Could you check a few things on this model? Use its own coordinates, in mm. Round coordinates to 2 decimals unless told otherwise and drop trailing zeros. Loops run counter-clockwise (first coordinate to the right, second up) from the corner with the lowest first, then second, coordinate; pieces in that order, holes last.
Autodesk Inventor part; units mm, degrees
ref_plane "YZ Plane" through (0, 0, 0) normal (1, 0, 0) x (0, 1, 0)
ref_plane "XZ Plane" through (0, 0, 0) normal (0, 1, 0) x (-1, 0, 0)
ref_plane "XY Plane" through (0, 0, 0) normal (0, 0, 1) x (1, 0, 0)
sketch "スケッチ3" plane through (0, 0, 0) normal (0, 0, 1) x (1, 0, 0)
  line L0 (60, -99.3436) -> (-60, -99.3436)
  line L1 (-60, -99.3436) -> (-60, 99.3436)
  line L2 (-60, 99.3436) -> (60, 99.3436)
  line L3 (60, 99.3436) -> (60, -99.3436)
  line L4 (60, -99.3436) -> (-60, 99.3436) construction
  line L5 (-60, -99.3436) -> (60, 99.3436) construction
  point P0 (0, 0)
  dimension "d25" = 120
extrude "押し出し1" add sketch "スケッチ3" against normal blind 3
sketch "スケッチ4" plane through (0, 0, 0) normal (0, 0, 1) x (1, 0, 0)
  line L0 (0, 45.0711) -> (68.3595, 45.0711)
  line L1 (68.3595, 45.0711) -> (-74.3824, 45.0711)
  line L2 (-74.3824, 45.0711) -> (108.1656, 45.0711)
  line L3 (108.1656, 45.0711) -> (108.1656, 129.4154)
  line L4 (108.1656, 129.4154) -> (-74.3824, 129.4154)
  line L5 (-74.3824, 129.4154) -> (-74.3824, 45.0711)
  point P0 (0, 0)
extrude "押し出し4" cut sketch "スケッチ4" against normal blind 10
sketch "スケッチ12" plane through (0, 0, 0) normal (0, 0, 1) x (1, 0, 0)
  circle A0 centre (0, 0) radius 7.5
  circle A1 centre (0, 0) radius 22.5
  dimension "d85" = 15
  dimension "d93" = 45
sketch "スケッチ13" plane through (0, 0, 0) normal (0, 0, 1) x (1, 0, 0)
  circle A0 centre (0, 0) radius 7.5
  circle A1 centre (0, 0) radius 32.5
  circle A2 centre (31.7707, 6.8465) radius 25
  circle A3 centre (31.7707, 6.8465) radius 7.5
  circle A4 centre (31.7707, 6.8465) radius 32.5
  circle A5 centre (28.5436, -25.4929) radius 25
  circle A6 centre (28.5436, -25.4929) radius 20
  circle A7 centre (28.5436, -25.4929) radius 60
  circle A8 centre (0, -78.2685) radius 40
  circle A9 centre (0, -78.2685) radius 50
  circle A10 centre (31.7707, 6.8465) radius 5
  circle A11 centre (28.5436, -25.4929) radius 9.5
  circle A12 centre (0, -78.2685) radius 9.5
  dimension "d87" = 65
  dimension "d89" = 65
  dimension "d91" = 120
  dimension "d86" = 15
  dimension "d88" = 15
  dimension "d90" = 40
  dimension "d92" = 100
  dimension "d96" = 10
  dimension "d97" = 19
  dimension "d98" = 19
extrude "押し出し15" cut sketch "スケッチ12" against normal blind 10 contours A0
extrude "押し出し16" cut sketch "スケッチ13" against normal blind 10 contours A10 A1 | A1 A10 | A11 A1 A2 | A2 A1 A4 A11 | A4 A1 A11 | A2 A11 A4 A1 | A1 A11 A2 | A4 A11 A1 | A12 A7 | A7 A12
sketch "スケッチ14" plane through (0, 0, 0) normal (0, 0, 1) x (1, 0, 0)
  line L0 (-60, -99.3436) -> (-60, 45.0711)
  line L1 (60, 45.0711) -> (60, -99.3436)
  line L2 (-60, 45.0711) -> (60, 45.0711)
  line L3 (60, 45.0711) -> (60, -92.9289)
  line L4 (60, -92.9289) -> (-60, -92.9289)
  line L5 (-60, -92.9289) -> (-60, 45.0711)
  point P0 (0, 0)
  dimension "d101" = 138
extrude "押し出し17" cut sketch "スケッチ14" against normal blind 10 keep common part
sketch "スケッチ15" plane through (-60, 45.0711, 0) normal (0, 1, 0) x (1, 0, 0)
  line L0 (-15.5399, 21.7204) -> (138.9638, 21.7204)
  line L1 (138.9638, 21.7204) -> (138.9638, -41.1938)
  line L2 (138.9638, -41.1938) -> (-15.5399, -41.1938)
  line L3 (-15.5399, -41.1938) -> (-15.5399, 21.7204)
  point P0 (60, 0)
extrude "押し出し18" cut sketch "スケッチ15" against normal blind 10
sketch "スケッチ16" plane through (0, 0, 0) normal (0, 0, 1) x (1, 0, 0)
  circle A0 centre (31.7707, 6.8465) radius 5
  circle A1 centre (31.7707, 6.8465) radius 25
  circle A2 centre (28.5436, -25.4929) radius 9.5
  circle A3 centre (28.5436, -25.4929) radius 25
  circle A4 centre (55, -13) radius 2
  circle A5 centre (-55, -13) radius 2
  circle A6 centre (0, 29) radius 2
  point P0 (0, 0)
  dimension "d109" = 50
  dimension "d110" = 50
  dimension "d111" = 4
  dimension "d112" = 4
  dimension "d113" = 4
extrude "押し出し19" cut sketch "スケッチ16" against normal blind 10 contours A4 | A5 | A6
sketch "スケッチ17" plane through (0, 0, 0) normal (0, 0, 1) x (1, 0, 0)
  line L0 (0, 0) -> (0, 14.5)
  line L1 (0, 14.5) -> (0, -14.5)
  circle A0 centre (0, 14.5) radius 2.15
  circle A1 centre (0, -14.5) radius 2.15
  dimension "d116" = 14.5
  dimension "d117" = 29
  dimension "d118" = 4.3
  dimension "d119" = 4.3
extrude "押し出し20" cut sketch "スケッチ17" against normal blind 10
properties part number "板2" material "アルミニウム 6061"
Item 1: If we section it at C-C, the plane x = 0: Please give me the cut outline in (y, z).
Results list:
outline: (-92.93, -3) - (-87.77, -3) - (-87.77, 0) - (-92.93, 0) - close; (-68.77, -3) - (-16.65, -3) - (-16.65, 0) - (-68.77, 0) - close; (-12.35, -3) - (-7.5, -3) - (-7.5, 0) - (-12.35, 0) - close; (7.5, -3) - (12.35, -3) - (12.35, 0) - (7.5, 0) - close; (16.65, -3) - (27, -3) - (27, 0) - (16.65, 0) - close; (31, -3) - (35.07, -3) - (35.07, 0) - (31, 0) - close
Item 2: We'd pull the mould along Y, two halves only. Please class faces 1 (the cylindrical face through (0, 27, -1)), 2 (the flat face through (60, -28, -1)), 3 (the flat face through (1, -92.929, -1)): released by +Y, released by -Y, zero draft, split by the parting line, or undercut.
Results list:
face 1: undercut
face 2: zero draft
face 3: released by -Y
Item 3: If we section it at D-D, the plane x = 29.5: Please give me the cut outline in (y, z), then the cut area to 3 significant figures.
Results list:
outline: (-92.93, -3) - (-34.94, -3) - (-34.94, 0) - (-92.93, 0) - close; (-16.04, -3) - (2.39, -3) - (2.39, 0) - (-16.04, 0) - close; (11.3, -3) - (35.07, -3) - (35.07, 0) - (11.3, 0) - close
area: 301 mm2
Item 4: If we section it at A-A, the plane y = 0: Please give me the cut outline in (x, z), then the cut area to 3 significant figures.
Results list:
outline: (-60, -3) - (-7.5, -3) - (-7.5, 0) - (-60, 0) - close; (7.5, -3) - (60, -3) - (60, 0) - (7.5, 0) - close
area: 315 mm2
Item 5: If we section it at B-B, the plane x = 55: Please give me the cut outline in (y, z), then the cut area to 3 significant figures.
Results list:
outline: (-92.93, -3) - (-15, -3) - (-15, 0) - (-92.93, 0) - close; (-11, -3) - (35.07, -3) - (35.07, 0) - (-11, 0) - close
area: 372 mm2
Item 6: If I drill on line 1 along Y through (x, z) = (0, -1.6); line 2 along Y through (x, z) = (-55, -2.25); line 3 along X through (y, z) = (-14.5, -1.6), over which ranges is the centre line in solid material (lowest first)?
Results list:
line 1: y = -92.93 to -87.77, -68.77 to -16.65, -12.35 to -7.5, 7.5 to 12.35, 16.65 to 27, 31 to 35.07
line 2: y = -92.93 to -15, -11 to 35.07
line 3: x = -60 to -56.32, -53.68 to -2.15, 2.15 to 53.68, 56.32 to 60
Item 7: Will this pin go through, and if not, where does the flat tip stop? pin 1 (4 mm diameter, centred on x = 0, y = 14.5, fed in from +Z).
Results list:
pin 1: passes through
